Model file for the job. Use its own axes, mm. Face numbers are marked on the shaded views. A direction names the side the tool comes from. Round coordinates to 2 decimals unless told otherwise and drop trailing zeros. Loops run counter-clockwise (first coordinate to the right, second up) from the corner with the lowest first, then second, coordinate; pieces in that order, holes last. Notation, with made-up numbers: M 37,9 L 44,9 A31 ccw 44,40 Z; hole C -17,2.5 d9. An arc over 180 degrees is marked long. Use a Markdown table: item, result. Add a question column.
Item 1: Pin check, flat tips, straight feed: P1, Ø14.5, axis at x = 131.96, y = 0, coming from the -Z side; P2, Ø1.5, axis at y = 1.5, z = 5.5, coming from the -X side; P3, Ø4, axis at x = 84, y = -1, coming from the -Z side; P4, Ø3, axis at x = 93, z = 9, coming from the +Y side. Stop position of each tip, or through.
Item 2: Tool access for the marked faces 1 and 2: list every direction of +Z, -Z, +X, -X, +Y, -Y with a clear straight run to the whole face (end or side of a thin tool).
Item 3: Wall check: L1, parallel to X at y = 0, z = 8.5; L2, parallel to X at y = 4.5, z = -0.25; L3, parallel to Y at x = 105, z = 0.5. Give the ranges that are in metal, low to high. Write a range as from..to.
Item 4: Saw through at A-A on x = 105.5. Write the cut outline in (y, z), then the cut area to 3 significant figures.
Item 5: Saw through at B-B on x = 16. Write the cut outline in (y, z), then the cut area to 3 significant figures.
```python
from build123d import *

# Parameters (mm, degrees)
SKETCH2_R               = 5.5
CUT_EXTRUDE1_DEPTH      = 13.5
CUT_EXTRUDE1_DEPTH_BACK = 13.5


with BuildPart() as part:
    # Sketch1 → Revolve1 (revolve)
    with BuildSketch(Plane.XY):
        Polygon((3.464101615, 6), (0, 0), (144.464101615, 0), (144.464101615, 10.5), (142.464101615, 12.5), (119.464101615, 12.5), (119.464101615, 10), (23.464101615, 10), (23.464101615, 6), (19.464101615, 6), (19.464101615, 4), (13.464101615, 4), (13.464101615, 6), align=None)
    revolve(axis=Axis((0, 0, 0), (1, 0, 0)))

    # Sketch2 → Cut-Extrude1 (cut, two sides)
    with BuildSketch(Plane.XY) as cut_extrude1_sk:
        with Locations((131.964101615, 0)):
            Circle(SKETCH2_R)
    extrude(amount=CUT_EXTRUDE1_DEPTH, mode=Mode.SUBTRACT)
    extrude(cut_extrude1_sk.sketch, amount=-CUT_EXTRUDE1_DEPTH_BACK, mode=Mode.SUBTRACT)


solid = part.part
```
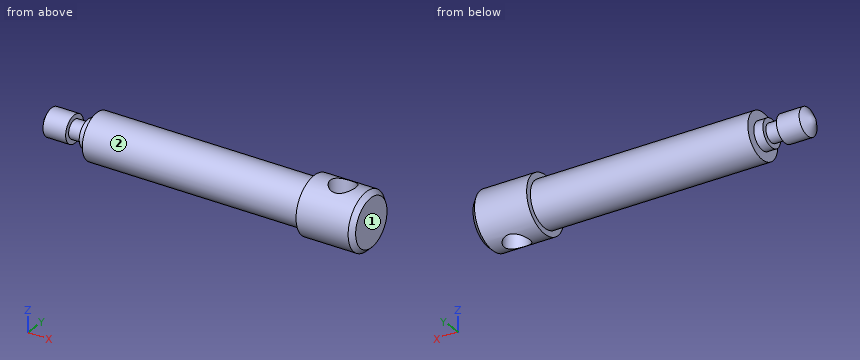
Entries:
| question | item | result |
|---|---|---|
| 1 | P1 | z = -12.5 |
| 1 | P2 | x = 2.86 |
| 1 | P3 | z = -10 |
| 1 | P4 | y = 6.61 |
| 2 | face 1 | +Z, -Z, +X, +Y, -Y |
| 2 | face 2 | -X |
| 3 | L1 | 23.46..126.46, 137.46..144.46 |
| 3 | L2 | 2.6..13.46, 19.46..128.8, 135.13..144.46 |
| 3 | L3 | -9.99..9.99 |
| 4 | outline | C 0,0 d20 |
| 4 | area | 314 mm2 |
| 5 | outline | C 0,0 d8 |
| 5 | area | 50.3 mm2 |
